Check sheet for the modelled part. Datum: model origin and axes. Units: mm. Round coordinates to 2 decimals unless told otherwise and drop trailing zeros. Write each loop counter-clockwise with the first axis right and the second up, starting at its lowest first coordinate (ties: lowest second). Pieces come first, ordered by that corner, then holes. Notation, with made-up numbers: M 3.5,17.5 L 38.5,17.5 A31 cw 38.5,46.5 Z; hole C 9,12 d10. An arc over 180 degrees is marked long. One line per item, written item: value.
from build123d import *

# Parameters (mm, degrees)
F0_W     = 8
F0_H     = 7.5
F1_DEPTH = 14
F3_R     = 0.75
F4_DEPTH = 8
F5_SIZE2 = 12
F5_SIZE  = 2
F6_R     = 2
F7_R     = 2


with BuildPart() as f1:
    # F0 (on Top) → F1 (new body)
    with BuildSketch(Plane.XY):
        Rectangle(F0_W, F0_H)
    extrude(amount=F1_DEPTH)

    # F3 (on face) → F4 (cut)
    with BuildSketch(Plane.YZ.offset(4)):
        with Locations((0, 3)):
            Circle(F3_R)
    extrude(amount=-F4_DEPTH, mode=Mode.SUBTRACT)

    # F5
    f5_edges = [f1.edges().sort_by_distance(p)[0] for p in [
        (0, -3.75, 0),
    ]]
    f5_side = f1.faces().sort_by_distance((0, 0, 0))[0]
    chamfer(f5_edges, length=F5_SIZE, length2=F5_SIZE2, reference=f5_side)

    # F6
    f6_edges = [f1.edges().sort_by_distance(p)[0] for p in [
        (0, -1.75, 0),
    ]]
    fillet(f6_edges, radius=F6_R)

    # F7
    f7_edges = [f1.edges().sort_by_distance(p)[0] for p in [
        (0, 3.75, 0),
    ]]
    fillet(f7_edges, radius=F7_R)


solid = f1.part
Q1. Sectioned sample at A-A on z = 3. Enter the section's corners in (x, y).
Completed:
outline: M -4,-2.25 L 4,-2.25 L 4,-0.75 L -4,-0.75 Z; M -4,0.75 L 4,0.75 L 4,3.75 L -4,3.75 Z
Q2. Sectioned sample at B-B on x = 0.25. Enter the section's corners in (y, z).
Completed:
outline: M -3.75,12 L -2.03,1.67 A2 ccw -0.06,0 L 1.75,0 A2 ccw 3.75,2 L 3.75,14 L -3.75,14 Z; hole C 0,3 d1.5
Q3. Scan lines: line 1 (Z direction, x = 0.75, y = 0); line 2 (Y direction, x = 0.5, z = 5.5); line 3 (Z direction, x = -1, y = 3). Record each from-to range of solid material in increasing order. Write a range as [from, to].
Completed:
line 1: [0, 2.25], [3.75, 14]
line 2: [-2.67, 3.75]
line 3: [0.44, 14]
Q4. Draft check along Z on faces 1 (the flat face through (0, -3.75, 13)), 2 (the cylindrical face through (0.056, -0.163, 2.268)), 3 (the flat face through (-0.1, -2.9, 6.9)). Enter one of: pulls with the +Z half, pulls with the -Z half, needs draft (parallel to the pull), parting line crosses it, or undercut.
Completed:
face 1: needs draft
face 2: undercut
face 3: pulls with the -Z half
Q5. Depth check by flat-ended pin: P1, Ø2, axis at x = -3, z = 2.5, coming from the -Y side. Enter the tip coordinate at first touch or a pass-through.
Completed:
P1: y = -2.33
Q6. Sectioned sample at C-C on y = -0.5. Enter the section's corners in (x, z), and give its area (3 significant figures).
Completed:
outline: M -4,0.05 L 4,0.05 L 4,2.44 L -4,2.44 Z; M -4,3.56 L 4,3.56 L 4,14 L -4,14 Z
area: 103 mm^2
Q7. Sectioned sample at D-D on z = 6.5. Enter the section's corners in (x, y).
Completed:
outline: M -4,-2.83 L 4,-2.83 L 4,3.75 L -4,3.75 Z
